from build123d import *

# Parameters (mm, degrees)
BOSS_EXTRUDE1_DEPTH = 38.1
SKETCH2_W           = 69.999999954
SKETCH2_H           = 90.000000086
CUT_EXTRUDE1_DEPTH  = 34.925
SKETCH3_R           = 3.96875
SKETCH3_R_2         = 1.5875
BOSS_EXTRUDE2_DEPTH = 11.43
BOSS_EXTRUDE3_DEPTH = 38.1
SKETCH5_R           = 1.5875
CUT_EXTRUDE2_DEPTH  = 12.7
SKETCH7_R           = 1.5875
CUT_EXTRUDE3_DEPTH  = 3.175


with BuildPart() as part:
    # Sketch1 → Boss-Extrude1 (new body)
    with BuildSketch(Plane(origin=(0, 0, 0), x_dir=(1, 0, 0), z_dir=(0, 1, 0))):
        with BuildLine():
            Line((3.175, 0), (73.174999954, 0))
            ThreePointArc((73.174999954, 0), (75.420063984, 0.92993597), (76.349999954, 3.175))
            Line((76.349999954, 3.175), (76.349999954, 93.175000086))
            ThreePointArc((76.349999954, 93.175000086), (75.420063984, 95.420064116), (73.174999954, 96.350000086))
            Line((73.174999954, 96.350000086), (3.175, 96.350000086))
            ThreePointArc((3.175, 96.350000086), (0.92993597, 95.420064116), (0, 93.175000086))
            Line((0, 93.175000086), (0, 3.175))
            ThreePointArc((0, 3.175), (0.92993597, 0.92993597), (3.175, 0))
        make_face()
    extrude(amount=BOSS_EXTRUDE1_DEPTH)

    # Sketch2 → Cut-Extrude1 (cut)
    with BuildSketch(Plane(origin=(0, 38.1, 0), x_dir=(1, 0, 0), z_dir=(0, 1, 0))):
        with Locations((38.174999977, 48.175000043)):
            Rectangle(SKETCH2_W, SKETCH2_H)
    extrude(amount=-CUT_EXTRUDE1_DEPTH, mode=Mode.SUBTRACT)

    # Sketch3 → Boss-Extrude2 (add)
    # profile 1 of 2: a face of its own
    with BuildSketch(Plane(origin=(0, 3.175, 0), x_dir=(1, 0, 0), z_dir=(0, 1, 0))):
        with Locations(Location((21.371999977, 88.775000043, 0), (0, 0, 90))):
            Circle(SKETCH3_R)
        with Locations(Location((21.371999977, 88.775000043, 0), (0, 0, 270))):
            Circle(SKETCH3_R_2, mode=Mode.SUBTRACT)
    # profile 2 of 2: a face of its own
    with BuildSketch(Plane(origin=(0, 3.175, 0), x_dir=(1, 0, 0), z_dir=(0, 1, 0))):
        with Locations(Location((39.704999977, 8.975000043, 0), (0, 0, 90))):
            Circle(SKETCH3_R)
        with Locations(Location((39.704999977, 8.975000043, 0), (0, 0, 270))):
            Circle(SKETCH3_R_2, mode=Mode.SUBTRACT)
    extrude(amount=BOSS_EXTRUDE2_DEPTH)

    # Sketch4 → Boss-Extrude3 (add)
    with BuildSketch(Plane.XZ):
        with BuildLine():
            Line((-6.35, -3.175), (-6.35, -93.175000086))
            ThreePointArc((-6.35, -93.175000086), (-3.560192091, -99.910192177), (3.175, -102.700000086))
            Line((3.175, -102.700000086), (73.174999954, -102.700000086))
            ThreePointArc((73.174999954, -102.700000086), (79.910192045, -99.910192177), (82.699999954, -93.175000086))
            Line((82.699999954, -93.175000086), (82.699999954, -3.175))
            ThreePointArc((82.699999954, -3.175), (79.910192045, 3.560192091), (73.174999954, 6.35))
            Line((73.174999954, 6.35), (3.175, 6.35))
            ThreePointArc((3.175, 6.35), (-3.560192091, 3.560192091), (-6.35, -3.175))
        make_face()
        with BuildLine():
            Line((0, -3.175), (0, -93.175000086))
            ThreePointArc((0, -93.175000086), (0.92993597, -95.420064116), (3.175, -96.350000086))
            Line((3.175, -96.350000086), (73.174999954, -96.350000086))
            ThreePointArc((73.174999954, -96.350000086), (75.420063984, -95.420064116), (76.349999954, -93.175000086))
            Line((76.349999954, -93.175000086), (76.349999954, -3.175))
            ThreePointArc((76.349999954, -3.175), (75.420063984, -0.92993597), (73.174999954, 0))
            Line((73.174999954, 0), (3.175, 0))
            ThreePointArc((3.175, 0), (0.92993597, -0.92993597), (0, -3.175))
        make_face(mode=Mode.SUBTRACT)
    extrude(amount=-BOSS_EXTRUDE3_DEPTH)

    # Sketch5 → Cut-Extrude2 (cut)
    with BuildSketch(Plane(origin=(0, 38.1, 0), x_dir=(1, 0, 0), z_dir=(0, 1, 0))):
        with Locations(Location((-1.5875, 48.175000043, 0), (0, 0, 270))):
            Circle(SKETCH5_R)
        with Locations(Location((38.174999977, 97.937500086, 0), (0, 0, 270))):
            Circle(SKETCH5_R)
        with Locations(Location((38.174999977, -1.5875, 0), (0, 0, 90))):
            Circle(SKETCH5_R)
        with Locations(Location((77.937499954, 48.175000043, 0), (0, 0, 90))):
            Circle(SKETCH5_R)
    extrude(amount=-CUT_EXTRUDE2_DEPTH, mode=Mode.SUBTRACT)

    # Sketch7 → Cut-Extrude3 (cut)
    with BuildSketch(Plane(origin=(0, 3.175, 0), x_dir=(1, 0, 0), z_dir=(0, 1, 0))):
        with Locations(Location((68.174999954, 70.175000043, 0), (0, 0, 270))):
            Circle(SKETCH7_R)
        with Locations(Location((68.174999954, 26.175000043, 0), (0, 0, 270))):
            Circle(SKETCH7_R)
    extrude(amount=-CUT_EXTRUDE3_DEPTH, mode=Mode.SUBTRACT)


solid = part.part
Check sheet for the modelled part. Datum: model origin and axes. Units: mm. A direction names the side the tool comes from. Give positions to 0.01 mm unless a question says otherwise; leave off trailing zeros. Loops run counter-clockwise (first coordinate to the right, second up) from the corner with the lowest first, then second, coordinate; pieces in that order, holes last. Notation, with made-up numbers: M 61,7 L 73,7 A31 ccw 73,41 Z; hole C -8.75,73.25 d11. An arc over 180 degrees is marked long. Return JSON: item names as keys, results as strings. Group by question number.
1. Cross-section at A-A on y = 9.5. State how many separate pieces and enclosed holes the cut face has, plus the area to 3 significant figures.
2. Thickness scan on L1, parallel to X at y = 30, z = -83 (3 decimals); L2, parallel to Z at x = 73, y = 11 (3 decimals); L3, parallel to Y at x = 41.5, z = -89 (3 decimals). Record the ranges inside material, lowest first.
3. Tool access check on faces 5 (the flat face through (2, 38.1, -52)), 6 (the cylindrical face through (-1.52, 31.84, -49.76)). Record the directions out of +Z, -Z, +X, -X, +Y, -Y that give a thin tool (end or side, any length) a straight path to the whole face; none if there is none.
4. Cross-section at B-B on z = -18. Record the boundary of the cut face in (x, y) (3 decimals).
5. Mould release check, pull along Z, two halves, no side actions. Record for faces 1 (the flat face through (38, 0, -47)), 2 (the flat face through (78, 25.4, -48)), 3 (the cylindrical face through (79.98, 18.78, 3.49)), 4 (the cylindrical face through (22.44, 8.81, -89.95)): released by +Z, released by -Z, zero draft, split by the parting line, or undercut.
6. Go/stop test with flat-tipped pins: pin 1 (3.5 mm diameter, centred on x = 39.5, z = -9, fed in from +Y) (3 decimals); pin 2 (1 mm diameter, centred on x = 38.5, z = -98.5, fed in from +Y); pin 3 (1 mm diameter, centred on x = 23, z = -84.5, fed in from +Y) (3 decimals). Record where each tip stops, or that it passes through.
7. Cross-section at C-C on x = 56. Record the boundary of the cut face in (y, z) (3 decimals).
Return value:
{
 "1": {"separate pieces": "3", "enclosed holes": "3", "area": "3,420 mm^2"},
 "2": {"L1": "-6.35 to 3.175, 73.175 to 82.7", "L2": "-102.7 to -93.175, -3.175 to 6.35", "L3": "0 to 3.175"},
 "3": {"face 5": "+Z, -Z, +X, -X, +Y", "face 6": "+Y"},
 "4": {"outline": "M -6.35,0 L 82.7,0 L 82.7,38.1 L 73.175,38.1 L 73.175,3.175 L 3.175,3.175 L 3.175,38.1 L -6.35,38.1 Z"},
 "5": {"face 1": "zero draft", "face 2": "undercut", "face 3": "released by +Z", "face 4": "undercut"},
 "6": {"pin 1": "y = 14.605", "pin 2": "y = 25.4", "pin 3": "y = 3.175"},
 "7": {"outline": "M 0,-102.7 L 38.1,-102.7 L 38.1,-93.175 L 3.175,-93.175 L 3.175,-3.175 L 38.1,-3.175 L 38.1,6.35 L 0,6.35 Z"}
}
